Geometry check sheet. Reference: the model listing, model coordinates, mm. Round coordinates to 2 decimals unless told otherwise and drop trailing zeros. Order: outer loops, then holes, each group sorted by start corner. A loop starts at its lowest first (then second) coordinate and runs counter-clockwise, first axis right, second up. Notation, with made-up numbers: (7, -26.75) -> (46, -26.75) arc R21 cw to (46, 4.25) -> close; hole circle Ø4 at (68, 53). An arc over 180 degrees is marked (long way). Answer as a JSON object with one key per item and string values. Group by question number.
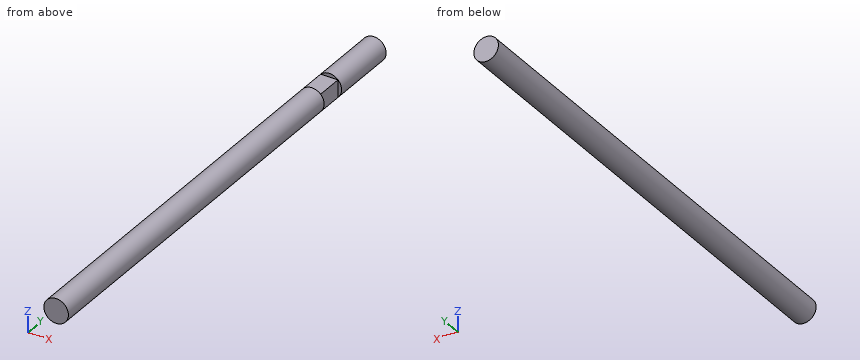
from build123d import *

# Parameters (mm, degrees)
CROQUIS1_R              = 2
SALIENTE_EXTRUIR1_DEPTH = 82
CORTAR_EXTRUIR1_DEPTH   = 4.5


with BuildPart() as part:
    # Croquis1 → Saliente-Extruir1 (new body)
    with BuildSketch(Plane(origin=(0, 0, 0), x_dir=(1, 0, 0), z_dir=(0, 1, 0))):
        with Locations(Location((0, 0, 0), (0, 0, 270))):
            Circle(CROQUIS1_R)
    extrude(amount=SALIENTE_EXTRUIR1_DEPTH)

    # Croquis2 → Cortar-Extruir1 (cut)
    with BuildSketch(Plane(origin=(0, 70.5, 0), x_dir=(1, 0, 0), z_dir=(0, 1, 0))):
        Polygon((2, -2), (-1.414213562, -2), (-1.414213562, -1.414213562), (1.414213562, -1.414213562), (1.414213562, 1.414213562), (2, 1.414213562), align=None)
    extrude(amount=-CORTAR_EXTRUIR1_DEPTH, mode=Mode.SUBTRACT)


solid = part.part
Item 1: Depth check by flat-ended pin: pin 1 Ø0.8 at (y, z) = (67, 0) entering from +X; pin 2 Ø1.4 at (x, y) = (-0.5, 69.5) entering from +Z. Enter the tip coordinate at first touch or a pass-through.
Item 2: Sectioned sample at A-A, the plane x = -0.75. Enter the section's corners in (y, z), then the cut area to 3 significant figures.
Item 3: Sectioned sample at B-B, the plane y = 52. Enter the section's corners in (x, z).
Item 4: Thickness scan on L1, parallel to Y at x = -0.8, z = 1.7; L2, parallel to X at y = 7.5, z = 0.2; L3, parallel to Z at x = -0.1, y = 60. Record the ranges inside material, lowest first.
Result:
{
 "1": {"pin 1": "stops at x = 1.41", "pin 2": "stops at z = 1.41"},
 "2": {"outline": "(0, -1.85) -> (82, -1.85) -> (82, 1.85) -> (70.5, 1.85) -> (70.5, 1.41) -> (66, 1.41) -> (66, 1.85) -> (0, 1.85) -> close", "area": "302 mm2"},
 "3": {"outline": "circle Ø4 at (0, 0)"},
 "4": {"L1": "y = 0 to 66, 70.5 to 82", "L2": "x = -1.99 to 1.99", "L3": "z = -2 to 2"}
}
